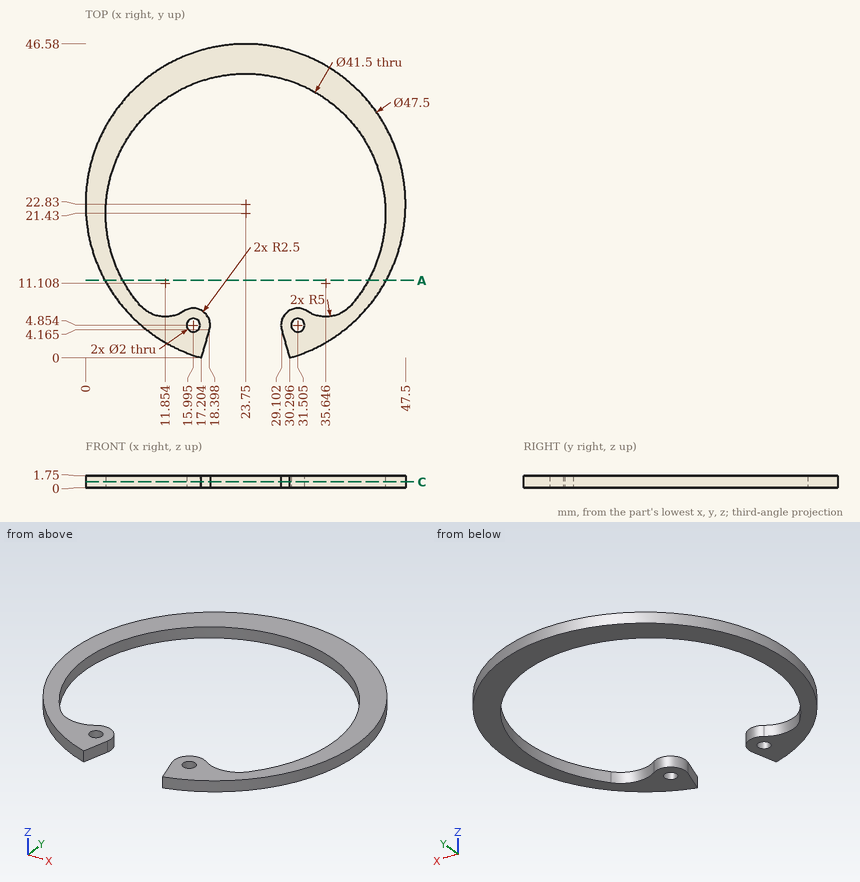
The figure shows three views and two pictorial views of one solid part (mm, origin at its lowest corner). Answer the questions. Give positions to 0.01 mm unless a question says otherwise; leave off trailing zeros. Loops run counter-clockwise (first coordinate to the right, second up) from the corner with the lowest first, then second, coordinate; pieces in that order, holes last. Notation, with made-up numbers: (23, 18) -> (79, 18) arc R22 cw to (79, 54) -> close; hole circle Ø2 at (77.25, -11.5). An arc over 180 degrees is marked (long way). Put each result on its own line as item: value. Start each with the question number.
Item 1: The part is cut by section A-A (y = 11.5). Give the vertices of the cut face in (x, z).
Item 2: The part is cut by section C-C (z = 0.85). State how many separate pieces and enclosed holes the cut face has.
Item 3: Find the intervals of material crossed by L1, parallel to X at y = 5, z = 1.2 (1 decimal); L2, parallel to Y at x = 31, z = 0.8 (1 decimal); L3, parallel to Y at x = 32, z = 0.25 (1 decimal), in increasing order. Write a range as [from, to].
Answers below:
1. outline: (2.88, 0) -> (5.53, 0) -> (5.53, 1.75) -> (2.88, 1.75) -> close; (41.97, 0) -> (44.62, 0) -> (44.62, 1.75) -> (41.97, 1.75) -> close
2. separate pieces: 1
2. enclosed holes: 2
3. L1: [8.1, 15], [17, 18.5], [29, 30.5], [32.5, 39.4]
3. L2: [0.2, 4], [5.7, 7.3], [40.9, 45.4]
3. L3: [0.6, 4], [5.7, 7.3], [40.5, 45.1]
